Read the model definition and answer for the solid it produces. Units are mm, in the model's axes. A direction names the side the tool comes from. Give positions to 0.01 mm unless a question says otherwise; leave off trailing zeros. Order: outer loops, then holes, each group sorted by start corner. A loop starts at its lowest first (then second) coordinate and runs counter-clockwise, first axis right, second up. Notation, with made-up numbers: M -33.75,41.25 L 24.25,41.25 A19 cw 24.25,68.25 Z; hole C 3.25,-2 d2. An arc over 180 degrees is marked long. One line per item, written item: value. Start each with the question number.
from build123d import *

# Parameters (mm, degrees)
SALIENTE_EXTRUIR1_DEPTH      = 25
SALIENTE_EXTRUIR1_DEPTH_BACK = 25
CROQUIS1_R                   = 5
REDONDEO9_R                  = 1
CORTAR_EXTRUIR1_DEPTH        = 49
CORTAR_EXTRUIR1_DEPTH_BACK   = 47
CROQUIS3_W                   = 70
CROQUIS3_H                   = 25
REDONDEO10_R                 = 20
CROQUIS4_R                   = 7.5
CORTAR_EXTRUIR2_DEPTH        = 65
REDONDEO11_R                 = 5


with BuildPart() as part:
    # Croquis1 → Saliente-Extruir1 (new, two sides: drawn at the far end of the back side and taken through both)
    with BuildSketch(Plane(origin=(0, 0, 0), x_dir=(1, 0, 0), z_dir=(0, 1, 0)).offset(-SALIENTE_EXTRUIR1_DEPTH_BACK)):
        with BuildLine():
            Line((-149.166666667, 24.986107251), (0.666666667, 19.988885801))
            ThreePointArc((0.666666667, 19.988885801), (20, 0), (0.666666667, -19.988885801))
            Line((0.666666667, -19.988885801), (-149.166666667, -24.986107251))
            ThreePointArc((-149.166666667, -24.986107251), (-175, 0), (-149.166666667, 24.986107251))
        make_face()
        with Locations(Location((-150, 0, 0), (0, 0, 270))):
            Circle(CROQUIS1_R, mode=Mode.SUBTRACT)
    extrude(amount=SALIENTE_EXTRUIR1_DEPTH + SALIENTE_EXTRUIR1_DEPTH_BACK)

    # Redondeo9
    redondeo9_edges = [part.edges().sort_by_distance(p)[0] for p in [
        (20, -25, 0),
        (-74.25, -25, -22.487496526),
        (-175, -25, 0),
        (-74.25, -25, 22.487496526),
    ]]
    fillet(redondeo9_edges, radius=REDONDEO9_R)

    # Croquis3 → Cortar-Extruir1 (cut, two sides: drawn at the far end of the back side and taken through both)
    with BuildSketch(Plane.XY.offset(-CORTAR_EXTRUIR1_DEPTH_BACK)):
        Rectangle(CROQUIS3_W, CROQUIS3_H)
    extrude(amount=CORTAR_EXTRUIR1_DEPTH + CORTAR_EXTRUIR1_DEPTH_BACK, mode=Mode.SUBTRACT)

    # Redondeo10
    redondeo10_edges = [part.edges().sort_by_distance(p)[0] for p in [
        (-35, 0, 21.178435734),
        (-35, 0, -21.178435734),
    ]]
    fillet(redondeo10_edges, radius=REDONDEO10_R)

    # Croquis4 → Cortar-Extruir2 (cut)
    with BuildSketch(Plane(origin=(0, 25, 0), x_dir=(1, 0, 0), z_dir=(0, 1, 0))):
        with Locations(Location((0, 0, 0), (0, 0, 270))):
            Circle(CROQUIS4_R)
    extrude(amount=-CORTAR_EXTRUIR2_DEPTH, mode=Mode.SUBTRACT)

    # Redondeo11
    redondeo11_edges = [part.edges().sort_by_distance(p)[0] for p in [
        (-175, 25, 0),
        (-74.25, 25, 22.487496526),
        (20, 25, 0),
        (-74.25, 25, -22.487496526),
    ]]
    fillet(redondeo11_edges, radius=REDONDEO11_R)


solid = part.part
Q1. Find section A-A, the plane z = 0. Give the vertices of the cut face in (x, y), then the cut area to 3 significant figures.
Q2. Find section D-D, the plane x = 2.5. State how many separate pieces and enclosed holes the cut face has, then the cut area to 3 significant figures.
Q3. Find section B-B, the plane y = 2. Give the vertices of the cut face in (x, z), then the cut area to 3 significant figures.
Q4. A tool of negligible diameter and unlimited length cuts with its end or side. For faces 4 (the cylindrical face through (-40.475, -0.175, 15.583)), 5 (the cylindrical face through (-73.249, 23.496, -21.028)), 6 (the cylindrical face through (-40.77, 0.18, -15.89)), from which of +Z, -Z, +X, -X, +Y, -Y can it reach the whole face along a straight path? Write none if from no direction.
Q5. Each of these flat-tipped pins is pushed along its axis until it touches: pin 1 (8 mm diameter, centred on y = 18.5, z = 20, fed in from -X); pin 2 (4 mm diameter, centred on x = -58, y = -5, fed in from +Z); pin 3 (1.8 mm diameter, centred on y = -5, z = -0.5, fed in from +X); pin 4 (6 mm diameter, centred on x = -150, z = 0, fed in from -Y). Where does it stop, or does it pass through?
Q6. Consider probe 1 along X at (y, z) = (15.25, 0); probe 2 along X at (y, z) = (0.5, 0); probe 3 along Y at (x, z) = (11.5, 4). Determine where each line is inside the solid, lowest interval first.
Q7. Determine the mould class of faces 1 (the cylindrical face through (0.33, 18.838, -7.493)), 2 (the flat face through (-18, -12.5, 0)), 3 (the flat face through (-35, 0, 0)) for opening direction X: released by +X, released by -X, zero draft, split by the parting line, or undercut.
Q8. Find section C-C, the plane y = -16. Give the vertices of the cut face in (x, z).
Evaluation:
1. outline: M -175,-24 A1 ccw -174,-25 L -155,-25 L -155,25 L -170,25 A5 ccw -175,20 Z; M -145,-25 L -7.5,-25 L -7.5,-12.5 L -35,-12.5 L -35,12.5 L -7.5,12.5 L -7.5,25 L -145,25 Z; M 7.5,-25 L 19,-25 A1 ccw 20,-24 L 20,-12.5 L 7.5,-12.5 Z; M 7.5,12.5 L 20,12.5 L 20,20 A5 ccw 15,25 L 7.5,25 Z
1. area: 7,490 mm2
2. separate pieces: 4
2. enclosed holes: 0
2. area: 627 mm2
3. outline: M -149.17,-24.99 L -54.33,-21.82 A20 ccw -35,-1.83 L -35,1.83 A20 ccw -54.33,21.82 L -149.17,24.99 A25 ccw long Z; hole C -150,0 d10
3. area: 6,060 mm2
4. face 4: +Z, +X
4. face 5: -Z, +X, +Y
4. face 6: -Z, +X
5. pin 1: x = -169.21
5. pin 2: z = 22.01
5. pin 3: x = -35
5. pin 4: through
6. probe 1: -175 to -155, -145 to -7.5, 7.5 to 20
6. probe 2: -175 to -155, -145 to -35
6. probe 3: -25 to -12.5, 12.5 to 25
7. face 1: undercut
7. face 2: zero draft
7. face 3: released by +X
8. outline: M -149.17,-24.99 L 0.67,-19.99 A20 ccw 0.67,19.99 L -149.17,24.99 A25 ccw long Z; hole C -150,0 d10; hole C 0,0 d15
